from build123d import *

# Parameters (mm, degrees)
SALIENTE_EXTRUIR1_DEPTH = 25
CROQUIS2_W              = 15
CROQUIS2_H              = 10
CROQUIS2_R              = 1.6
SALIENTE_EXTRUIR2_DEPTH = 3
CROQUIS3_W              = 10
CROQUIS3_H              = 4
CORTAR_EXTRUIR1_DEPTH   = 33


with BuildPart() as part:
    # Croquis1 → Saliente-Extruir1 (new body)
    with BuildSketch(Plane.XY):
        Polygon((15.9, 5.5), (14.4, 1.5), (25.6, 1.5), (24.1, 5.5), (40, 5.5), (40, 0), (0, 0), (0, 5.5), align=None)
    extrude(amount=SALIENTE_EXTRUIR1_DEPTH)

    # Croquis2 → Saliente-Extruir2 (add)
    with BuildSketch(Plane.XY.offset(25)):
        with Locations((20, 5)):
            Rectangle(CROQUIS2_W, CROQUIS2_H)
        with Locations((20, 5.5)):
            Circle(CROQUIS2_R, mode=Mode.SUBTRACT)
    extrude(amount=-SALIENTE_EXTRUIR2_DEPTH)

    # Croquis3 → Cortar-Extruir1 (cut)
    with BuildSketch(Plane.XY.offset(25)):
        with Locations((5, 3.5)):
            Rectangle(CROQUIS3_W, CROQUIS3_H)
        with Locations((35, 3.5)):
            Rectangle(CROQUIS3_W, CROQUIS3_H)
    extrude(amount=-CORTAR_EXTRUIR1_DEPTH, mode=Mode.SUBTRACT)


solid = part.part
Geometry check sheet. Reference: the model listing, model coordinates, mm. A direction names the side the tool comes from. Give positions to 0.01 mm unless a question says otherwise; leave off trailing zeros. Order: outer loops, then holes, each group sorted by start corner. A loop starts at its lowest first (then second) coordinate and runs counter-clockwise, first axis right, second up.
1. Access from +Z, -Z, +X, -X, +Y, -Y to the whole of each face (thin tool, end or side, straight path). Record for faces 1 (the face through (27.5, 8, 24)), 2 (the face through (12.5, 8, 24)), 3 (the face through (20, 1.5, 11)), 4 (the face through (0, 1, 12)), 5 (the face through (18.73, 4.53, 23.52)).
Completed:
face 1: +Z, -Z, +X, +Y
face 2: +Z, -Z, -X, +Y
face 3: -Z
face 4: +Z, -Z, -X, +Y, -Y
face 5: +Z, -Z
2. Sectioned sample at A-A (z = 22.5). Record the boundary of the cut face in (x, y), then the cut area to 3 significant figures.
Completed:
outline: (0, 0) - (40, 0) - (40, 1.5) - (30, 1.5) - (30, 5.5) - (27.5, 5.5) - (27.5, 10) - (12.5, 10) - (12.5, 5.5) - (10, 5.5) - (10, 1.5) - (0, 1.5) - close; hole circle Ø3.2 at (20, 5.5)
area: 199 mm2
3. Sectioned sample at B-B (x = 20). Record the boundary of the cut face in (y, z), then the cut area to 3 significant figures.
Completed:
outline: (0, 0) - (1.5, 0) - (1.5, 22) - (3.9, 22) - (3.9, 25) - (0, 25) - close; (7.1, 22) - (10, 22) - (10, 25) - (7.1, 25) - close
area: 53.4 mm2
4. Sectioned sample at D-D (y = 7.5). Record the boundary of the cut face in (x, z), then the cut area to 3 significant figures.
Completed:
outline: (12.5, 22) - (27.5, 22) - (27.5, 25) - (12.5, 25) - close
area: 45.0 mm2
5. Sectioned sample at C-C (z = 8.5). Record the boundary of the cut face in (x, y), then the cut area to 3 significant figures.
Completed:
outline: (0, 0) - (40, 0) - (40, 1.5) - (30, 1.5) - (30, 5.5) - (24.1, 5.5) - (25.6, 1.5) - (14.4, 1.5) - (15.9, 5.5) - (10, 5.5) - (10, 1.5) - (0, 1.5) - close
area: 101 mm2
6. Draft check along Y on faces 6 (the face through (24.86, 3.47, 10.85)), 7 (the face through (20, 10, 24)), 8 (the face through (20, 3, 25)). Enter one of: pulls with the +Y half, pulls with the -Y half, needs draft (parallel to the pull), parting line crosses it, or undercut.
Completed:
face 6: undercut
face 7: pulls with the +Y half
face 8: needs draft
7. Depth check by flat-ended pin: pin 1 (4.5 mm diameter, centred on x = 13, z = 8.5, fed in from +Y); pin 2 (5 mm diameter, centred on x = 20, y = 5.5, fed in from -Z); pin 3 (2 mm diameter, centred on y = 4, z = 16.5, fed in from -X); pin 4 (3 mm diameter, centred on x = 8, y = 2.5, fed in from -Z). Enter the tip coordinate at first touch or a pass-through.
Completed:
pin 1: stops at y = 5.5
pin 2: stops at z = 22
pin 3: stops at x = 10
pin 4: stops at z = 0
8. Scan lines: line 1 (Y direction, x = 20, z = 24.4); line 2 (Y direction, x = 24, z = 10.75); line 3 (Z direction, x = 19, y = 3). Record each from-to range of solid material in increasing order.
Completed:
line 1: y = 0 to 3.9, 7.1 to 10
line 2: y = 0 to 1.5
line 3: z = 22 to 25
